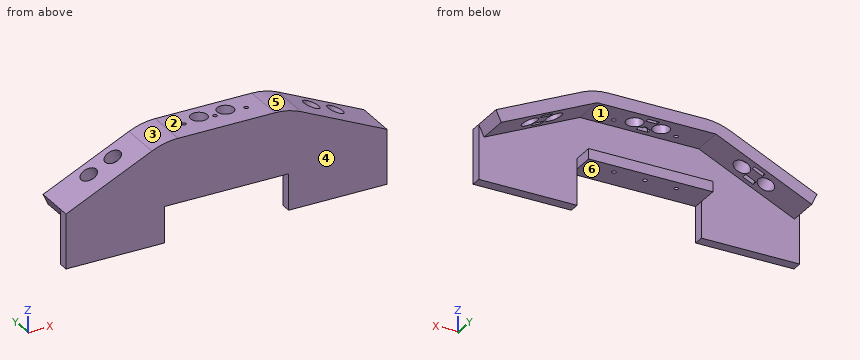
from build123d import *

# Parameters (mm, degrees)
EXTRUDE_THIN1_DEPTH = 30
SKETCH2_R           = 8
CUT_EXTRUDE1_DEPTH  = 141.868386798
SKETCH3_R           = 8
CUT_EXTRUDE2_DEPTH  = 56.174920969
BOSS_EXTRUDE1_DEPTH = 10
SKETCH7_W           = 120
SKETCH7_H           = 30
BOSS_EXTRUDE2_DEPTH = 10
SKETCH8_R           = 2
CUT_EXTRUDE3_DEPTH  = 63
FILLET1_R           = 60
SKETCH9_W           = 95
SKETCH9_H           = 52.700772475
BOSS_EXTRUDE3_DEPTH = 10
SKETCH10_W          = 11
SKETCH10_H          = 4
SKETCH10_H_2        = 5
CUT_EXTRUDE4_DEPTH  = 4.5
SKETCH13_W          = 11
SKETCH13_H          = 5
SKETCH13_H_2        = 4
CUT_EXTRUDE5_DEPTH  = 4


with BuildPart() as part:
    # Sketch1 → Extrude-Thin1 (new body)
    with BuildSketch(Plane(origin=(0, 0, 0), x_dir=(1, 0, 0), z_dir=(0, 1, 0))):
        Polygon((-155, 44.299227525), (-60, 0), (60, 0), (155, 44.299227525), (149.928580859, 55.174920969), (57.339664048, 12), (-57.339664048, 12), (-149.928580859, 55.174920969), align=None)
    extrude(amount=EXTRUDE_THIN1_DEPTH)

    # Sketch2 → Cut-Extrude1 (cut, through all)
    with BuildSketch(Plane(origin=(10.716371709, 0, 22.981333294), x_dir=(0.906307787, 0, -0.422618262), z_dir=(0.422618262, 0, 0.906307787))):
        with Locations((93.988918373, 15)):
            Circle(SKETCH2_R)
        with Locations((119.588918373, 15)):
            Circle(SKETCH2_R)
    cut_extrude1 = extrude(amount=-CUT_EXTRUDE1_DEPTH, mode=Mode.SUBTRACT)

    # Mirror1: Cut-Extrude1 across plane
    add(cut_extrude1.mirror(Plane(origin=(0, 0, 0), x_dir=(0, 0, 1), z_dir=(1, 0, 0))), mode=Mode.SUBTRACT)

    # Sketch3 → Cut-Extrude2 (cut, through all)
    with BuildSketch(Plane.XY):
        with Locations((12.8, 15)):
            Circle(SKETCH3_R)
        with Locations((-12.8, 15)):
            Circle(SKETCH3_R)
    extrude(amount=-CUT_EXTRUDE2_DEPTH, mode=Mode.SUBTRACT)

    # Sketch5 → Boss-Extrude1 (add)
    with BuildSketch(Plane.XZ):
        Polygon((66.80863999, -55.174920969), (149.928580859, -55.174920969), (57.339664048, -12), (-57.339664048, -12), (-149.928580859, -55.174920969), (-66.80863999, -55.174920969), (-60, -52), (60, -52), align=None)
        Polygon((-155, -44.299227525), (-149.928580859, -55.174920969), (-57.339664048, -12), (57.339664048, -12), (149.928580859, -55.174920969), (155, -44.299227525), (60, 0), (-60, 0), align=None)
    extrude(amount=BOSS_EXTRUDE1_DEPTH)

    # Sketch7 → Boss-Extrude2 (add)
    with BuildSketch(Plane(origin=(0, 0, -52), x_dir=(-1, 0, 0), z_dir=(0, 0, -1))):
        with Locations((0, 5)):
            Rectangle(SKETCH7_W, SKETCH7_H)
    extrude(amount=BOSS_EXTRUDE2_DEPTH)

    # Sketch8 → Cut-Extrude3 (cut, through all)
    with BuildSketch(Plane(origin=(0, 0, -62), x_dir=(-1, 0, 0), z_dir=(0, 0, -1))):
        with Locations((0, 10)):
            Circle(SKETCH8_R)
        with Locations((-30, 10)):
            Circle(SKETCH8_R)
        with Locations((30, 10)):
            Circle(SKETCH8_R)
    extrude(amount=-CUT_EXTRUDE3_DEPTH, mode=Mode.SUBTRACT)

    # Fillet1
    fillet1_edges = [part.edges().sort_by_distance(p)[0] for p in [
        (60, 10, 0),
        (-60, 10, 0),
    ]]
    fillet(fillet1_edges, radius=FILLET1_R)

    # Sketch9 → Boss-Extrude3 (add)
    with BuildSketch(Plane(origin=(0, 0, 0), x_dir=(1, 0, 0), z_dir=(0, 1, 0))):
        with Locations((107.5, 70.649613762)):
            Rectangle(SKETCH9_W, SKETCH9_H)
    boss_extrude3 = extrude(amount=-BOSS_EXTRUDE3_DEPTH)

    # Mirror2: Boss-Extrude3 across plane
    add(boss_extrude3.mirror(Plane(origin=(0, 0, 0), x_dir=(0, 0, 1), z_dir=(1, 0, 0))))

    # Sketch10 → Cut-Extrude4 (cut)
    with BuildSketch(Plane(origin=(5.644952569, 0, 12.105639849), x_dir=(-0.906307787, 0, 0.422618262), z_dir=(-0.422618262, 0, -0.906307787))):
        with Locations((-106.788918373, 23.3)):
            Rectangle(SKETCH10_W, SKETCH10_H)
        with Locations((-106.788918373, 7.2)):
            Rectangle(SKETCH10_W, SKETCH10_H_2)
    cut_extrude4 = extrude(amount=-CUT_EXTRUDE4_DEPTH, mode=Mode.SUBTRACT)

    # Mirror3: Cut-Extrude4 across plane
    add(cut_extrude4.mirror(Plane(origin=(0, 0, 0), x_dir=(0, 0, 1), z_dir=(1, 0, 0))), mode=Mode.SUBTRACT)

    # Sketch13 → Cut-Extrude5 (cut)
    with BuildSketch(Plane(origin=(0, 0, -12), x_dir=(-1, 0, 0), z_dir=(0, 0, -1))):
        with Locations((0, 7.2)):
            Rectangle(SKETCH13_W, SKETCH13_H)
        with Locations((0, 23.3)):
            Rectangle(SKETCH13_W, SKETCH13_H_2)
    extrude(amount=-CUT_EXTRUDE5_DEPTH, mode=Mode.SUBTRACT)


solid = part.part
Design review of the part built by this model. Coordinates are the model's own, in mm. Face numbers are marked on the shaded views. A direction names the side the tool comes from. Round coordinates to 2 decimals unless told otherwise and drop trailing zeros. Write each loop counter-clockwise with the first axis right and the second up, starting at its lowest first coordinate (ties: lowest second). Pieces come first, ordered by that corner, then holes. Notation, with made-up numbers: (76.25, 14.5) - (119.25, 14.5) arc R25 cw to (119.25, 53.5) - close; hole circle Ø7 at (14.5, 56.25). An arc over 180 degrees is marked (long way). Return JSON: item names as keys, results as strings. Group by question number.
Item 1: The part is to be moulded in two halves that separate along X. For the marked faces 3, 4, 5 and 6, say which applies: pulls with the +X half, pulls with the -X half, needs draft (parallel to the pull), parting line crosses it, or undercut.
Item 2: We need section A-A on x = 12.8. Write out the cut boundary in (y, z).
Item 3: We need section B-B on y = -4. Write out the cut boundary in (x, z).
Item 4: Machinability: for the marked faces 1 and 2, which of the approach directions +Z, -Z, +X, -X, +Y, -Y give a long, thin tool a straight path to every point of the face, cutting with its end or side? Answer none if there is none.
Item 5: We need section C-C on x = -52.5. Write out the cut boundary in (y, z).
Item 6: For probe 1 along Y at (x, z) = (0, -4); probe 2 along X at (y, z) = (-3, -75); probe 3 along Z at (x, y) = (10.5, 5), list the stretches that pass through material, from the lowest coordinate up. Write a range as [from, to].
Item 7: We need section D-D on y = 15. Give the number of separate pieces and of enclosed holes in the cut face, and give its area (3 significant figures).
Item 8: Insertion check: P1, Ø1.2, axis at y = 6.5, z = -10.5, coming from the -X side; P2, Ø3, axis at x = 0, y = 10, coming from the +Z side; P3, Ø6, axis at x = -1.5, z = -16.5, coming from the +Y side; P4, Ø6, axis at x = 45, y = 4, coming from the -Z side. Each pin has a flat end and moves straight along its axis. Give the tip position at first contact, or say it passes through.
Model answer:
{
 "1": {"face 3": "pulls with the -X half", "face 4": "needs draft", "face 5": "pulls with the +X half", "face 6": "undercut"},
 "2": {"outline": "(-10, -62) - (20, -62) - (20, -52) - (0, -52) - (0, -12) - (7, -12) - (7, 0) - (-10, 0) - close; (23, -12) - (30, -12) - (30, 0) - (23, 0) - close"},
 "3": {"outline": "(-155, -97) - (-60, -97) - (-60, -62) - (60, -62) - (60, -97) - (155, -97) - (155, -44.3) - (72.06, -5.62) arc R60 ccw to (46.7, 0) - (-46.7, 0) arc R60 ccw to (-72.06, -5.62) - (-155, -44.3) - close"},
 "4": {"face 1": "+Y", "face 2": "+Z, +X, -X, +Y, -Y"},
 "5": {"outline": "(-10, -62) - (20, -62) - (20, -52) - (0, -52) - (0, -12) - (30, -12) - (30, -0.28) - (-10, -0.28) - close"},
 "6": {"probe 1": "y = [-10, 8], [12, 30]", "probe 2": "x = [-155, -60], [60, 155]", "probe 3": "z = [-62, -52], [-12, 0]"},
 "7": {"separate pieces": "8", "enclosed holes": "0", "area": "3,910 mm²"},
 "8": {"P1": "stops at x = -83.8", "P2": "passes through", "P3": "stops at y = 0", "P4": "stops at z = -62"}
}
